```python
from build123d import *

# Parameters (mm, degrees)
SKETCH_1_R           = 2.75
EXTRUDE_1_DEPTH      = 5
SKETCH_2_R           = 4.250000000000005
EXTRUDE_2_DEPTH      = 5
SKETCH_3_R           = 2.250000000000002
CUT_EXTRUDE_1_DEPTH  = 40.00000000000001
HOLE_WIZARD_M1_8_1_D = 2.1
SKETCH_8_R           = 7.499999999835785
SKETCH_8_R_2         = 2.249999999836049
EXTRUDE_3_DEPTH      = 1


with BuildPart() as part:
    # 스케치1 → 보스-돌출1 (new body)
    with BuildSketch(Plane.XY):
        with BuildLine():
            Line((2.51e-15, 10.5), (30, 7.5))
            ThreePointArc((30, 7.5), (37.5, 0), (30, -7.5))
            Line((30, -7.5), (2.51e-15, -10.5))
            ThreePointArc((2.51e-15, -10.5), (-10.5, 1.29e-15), (2.51e-15, 10.5))
        make_face()
        Circle(SKETCH_1_R, mode=Mode.SUBTRACT)
    extrude(amount=EXTRUDE_1_DEPTH)

    # 스케치2 → 보스-돌출2 (add)
    with BuildSketch(Plane.XY.offset(5)):
        with Locations((30, 0)):
            Circle(SKETCH_2_R)
    extrude(amount=EXTRUDE_2_DEPTH)

    # 스케치3 → 컷-돌출1 (cut)
    with BuildSketch(Plane.XY.offset(10)):
        with Locations((30, 0)):
            Circle(SKETCH_3_R)
    extrude(amount=-CUT_EXTRUDE_1_DEPTH, mode=Mode.SUBTRACT)

    # M1.8 여유 구멍1 (through all)
    with Locations(Plane(origin=(0, 0, 0), x_dir=(-1, 0, 0), z_dir=(0, 0, -1))):
        with Locations((-7.172291773, -3.251754556), (3.251754556, -7.172291774), (7.172291774, 3.251754554), (-3.251754555, 7.172291773)):
            Hole(HOLE_WIZARD_M1_8_1_D / 2)

    # 스케치8 → 보스-돌출3 (add)
    with BuildSketch(Plane.XY.offset(5)):
        with Locations(Location((30.000000000162284, 3.18634e-11, 0), (0, 0, 269.999999996))):
            Circle(SKETCH_8_R)
        with Locations((30.000000000162284, 3.18634e-11)):
            Circle(SKETCH_8_R_2, mode=Mode.SUBTRACT)
    extrude(amount=EXTRUDE_3_DEPTH)


solid = part.part
```
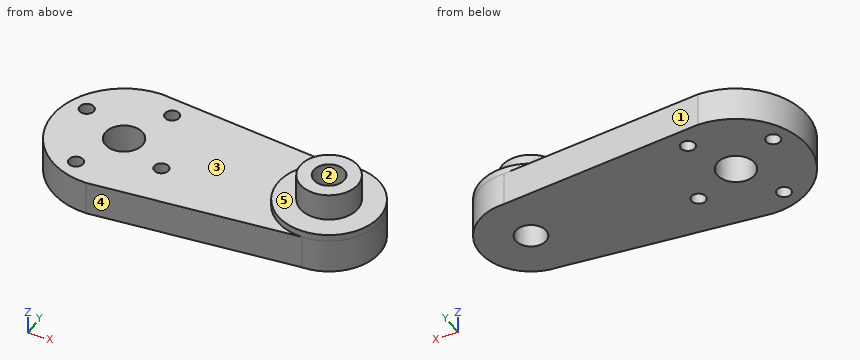
Source: CAD feature listing. Evaluate the final solid. Frame: model axes, mm. Face numbers are marked on the shaded views. A direction names the side the tool comes from. Give positions to 0.01 mm unless a question says otherwise; leave off trailing zeros. Loops run counter-clockwise (first coordinate to the right, second up) from the corner with the lowest first, then second, coordinate; pieces in that order, holes last. Notation, with made-up numbers: (54, 15.5) - (59, 15.5) arc R34 ccw to (59, 52.5) - close; hole circle Ø7 at (69, 80). An arc over 180 degrees is marked (long way). Use CSV: the item, a comma, the result in double quotes.
1) Cut plane C-C (z = 3.75). Output: boundary loops of the cut face in (x, y), and give its area (3 significant figures).
Worked out:
outline,"(0, -10.5) - (30, -7.5) arc R7.5 ccw to (30, 7.5) - (0, 10.5) arc R10.5 ccw to start; hole circle Ø2.1 at (-7.17, 3.25); hole circle Ø2.1 at (-3.25, -7.17); hole circle Ø5.5 at (0, 0); hole circle Ø2.1 at (3.25, 7.17); hole circle Ø2.1 at (7.17, -3.25); hole circle Ø4.5 at (30, 0)"
area,"748 mm^2"
2) Line query: line 1 (X direction, y = 2.5, z = 4.75); line 2 (Z direction, x = 9, y = -2.5); line 3 (X direction, y = 0.75, z = 3.5). Output: solid intervals per line, ascending.
Worked out:
line 1,"x = -10.2 to -7.91, -6.44 to -1.15, 1.15 to 37.07"
line 2,"z = 0 to 5"
line 3,"x = -10.47 to -2.65, 2.65 to 27.88, 32.12 to 37.46"
3) Mould query, pull axis X, two halves, no side actions, for the marked faces 1, 2 and 3. Classes: +X half, -X half, draft (parallel to the pull), parting line (faces both ways), or undercut.
Worked out:
face 1,"+X half"
face 2,"undercut"
face 3,"draft"
4) Cut plane A-A (y = 0). Output: boundary loops of the cut face in (x, z).
Worked out:
outline,"(-10.5, 0) - (-2.75, 0) - (-2.75, 5) - (-10.5, 5) - close; (2.75, 0) - (27.75, 0) - (27.75, 10) - (25.75, 10) - (25.75, 6) - (22.5, 6) - (22.5, 5) - (2.75, 5) - close; (32.25, 0) - (37.5, 0) - (37.5, 6) - (34.25, 6) - (34.25, 10) - (32.25, 10) - close"
5) Set-up query: the marked faces 4 and 5. Return all of +Z, -Z, +X, -X, +Y, -Y with unobstructed straight access to the full face (end or side cutting, diameter ignored); none if empty.
Worked out:
face 4,"+Z, -Z, +X, -Y"
face 5,"+Z"
6) Cut plane D-D (z = 9). Output: boundary loops of the cut face in (x, y), and give its area (3 significant figures).
Worked out:
outline,"circle Ø8.5 at (30, 0); hole circle Ø4.5 at (30, 0)"
area,"40.8 mm^2"
7) Pin query (flat end, axial travel): P1, Ø4, axis at x = 32, z = 7, coming from the -Y side; P2, Ø5, axis at y = 5, z = 6, coming from the +X side; P3, Ø12, axis at x = 9, y = -5, coming from the +Z side. Return the tip coordinate at first contact, or that it passes through.
Worked out:
P1,"stops at y = -7.5"
P2,"stops at x = 37.07"
P3,"stops at z = 5"
8) Cut plane B-B (x = 29.5). Output: boundary loops of the cut face in (y, z).
Worked out:
outline,"(-7.55, 0) - (-2.19, 0) - (-2.19, 10) - (-4.22, 10) - (-4.22, 6) - (-7.48, 6) - (-7.48, 5) - (-7.55, 5) - close; (2.19, 0) - (7.55, 0) - (7.55, 5) - (7.48, 5) - (7.48, 6) - (4.22, 6) - (4.22, 10) - (2.19, 10) - close"
